from build123d import *

# Parameters (mm, degrees)
F0_W     = 996
F0_H     = 2210
F1_DEPTH = 160
F2_R     = 100
F3_R     = 200
F5_DEPTH = 160


with BuildPart() as f1:
    # F0 (on Top) → F1 (new body)
    with BuildSketch(Plane.XY):
        with Locations((440.006502, 1048.075508)):
            Rectangle(F0_W, F0_H)
    extrude(amount=F1_DEPTH)

    # F2
    f2_edges = [f1.edges().sort_by_distance(p)[0] for p in [
        (938.006502, 2153.075508, 80),
    ]]
    fillet(f2_edges, radius=F2_R)

    # F3
    f3_edges = [f1.edges().sort_by_distance(p)[0] for p in [
        (938.006502, -56.924492, 80),
    ]]
    fillet(f3_edges, radius=F3_R)

    # F4 (on face) → F5 (cut, through all)
    with BuildSketch(Plane.XY.offset(160)):
        with BuildLine():
            Line((672.006502, 2013.075508), (212.006502, 2013.075508))
            ThreePointArc((212.006502, 2013.075508), (141.295824, 1983.786186), (112.006502, 1913.075508))
            Line((112.006502, 1913.075508), (112.006502, 1063.075508))
            ThreePointArc((112.006502, 1063.075508), (141.295824, 992.36483), (212.006502, 963.075508))
            Line((212.006502, 963.075508), (672.006502, 963.075508))
            ThreePointArc((672.006502, 963.075508), (742.71718, 992.36483), (772.006502, 1063.075508))
            Line((772.006502, 1063.075508), (772.006502, 1913.075508))
            ThreePointArc((772.006502, 1913.075508), (742.71718, 1983.786186), (672.006502, 2013.075508))
        make_face()
    extrude(amount=-F5_DEPTH, mode=Mode.SUBTRACT)


solid = f1.part
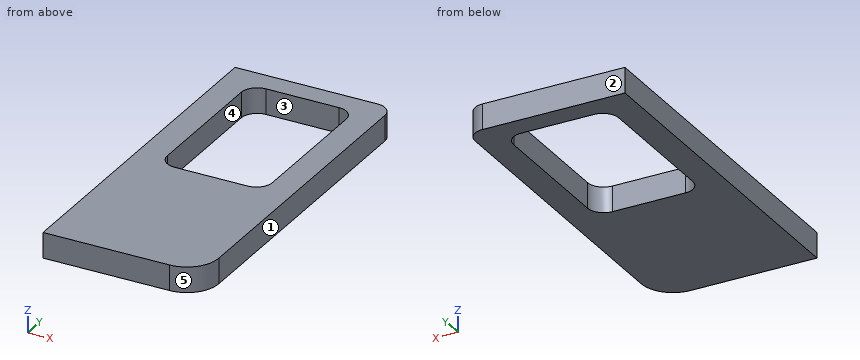
Read the model definition and answer for the solid it produces. Units are mm, in the model's axes. Face numbers are marked on the shaded views. A direction names the side the tool comes from. Round coordinates to 2 decimals unless told otherwise and drop trailing zeros. Write each loop counter-clockwise with the first axis right and the second up, starting at its lowest first coordinate (ties: lowest second). Pieces come first, ordered by that corner, then holes.
1. The part is cut by section B-B, the plane y = 1168. Determine the outline of the cut face in (x, z), then the cut area to 3 significant figures.
2. The part is cut by section A-A, the plane x = 359. Determine the outline of the cut face in (y, z).
3. The part is cut by section C-C, the plane z = 135.5. Determine the outline of the cut face in (x, y), then the cut area to 3 significant figures.
4. Straight lines are drawn through the part: L1, parallel to X at y = 1475.5, z = 76; L2, parallel to Y at x = 426.5, z = 58.5; L3, parallel to Y at x = 183, z = 131.5. For each, find the intervals that lie inside material, in ascending order.
5. Determine the mould class of the marked faces 1, 2 and 3 for opening direction Y: pulls with the +Y half, pulls with the -Y half, needs draft (parallel to the pull), parting line crosses it, or undercut.
6. Given pin 1 Ø8 at (x, z) = (758.5, 119.5) entering from -Y, flat-ended and moving along its own axis, determine where the tip first touches the part or whether it passes through.
7. Which of the six approach directions +Z, -Z, +X, -X, +Y, -Y give full straight-line access (tool end or side, diameter ignored) to the marked faces 4 and 5?
Values:
1. outline: (-57.99, 0) - (112.01, 0) - (112.01, 160) - (-57.99, 160) - close; (772.01, 0) - (938.01, 0) - (938.01, 160) - (772.01, 160) - close
1. area: 53,800 mm2
2. outline: (-56.92, 0) - (963.08, 0) - (963.08, 160) - (-56.92, 160) - close; (2013.08, 0) - (2153.08, 0) - (2153.08, 160) - (2013.08, 160) - close
3. outline: (-57.99, -56.92) - (738.01, -56.92) arc R200 ccw to (938.01, 143.08) - (938.01, 2053.08) arc R100 ccw to (838.01, 2153.08) - (-57.99, 2153.08) - close; hole (112.01, 1063.08) arc R100 ccw to (212.01, 963.08) - (672.01, 963.08) arc R100 ccw to (772.01, 1063.08) - (772.01, 1913.08) arc R100 ccw to (672.01, 2013.08) - (212.01, 2013.08) arc R100 ccw to (112.01, 1913.08) - close
3. area: 1,510,000 mm2
4. L1: x = -57.99 to 112.01, 772.01 to 938.01
4. L2: y = -56.92 to 963.08, 2013.08 to 2153.08
4. L3: y = -56.92 to 967.37, 2008.78 to 2153.08
5. face 1: needs draft
5. face 2: pulls with the +Y half
5. face 3: undercut
6. pin 1: stops at y = -56.24
7. face 4: +Z, -Z
7. face 5: +Z, -Z, +X, -Y
